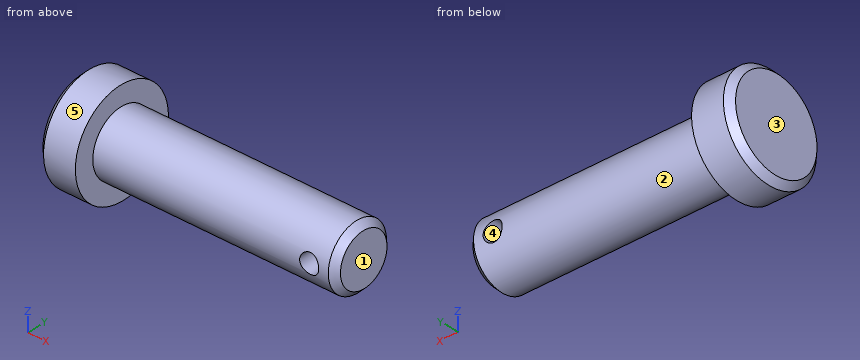
```python
from build123d import *

# Parameters (mm, degrees)
CHAMFER_1_SIZE           = 1
CHAMFER_2_SIZE           = 1
CUT_EXTRUDE_2_DEPTH      = 29.599611497
CUT_EXTRUDE_2_DEPTH_BACK = 29.599611497
SKETCH_2_R               = 1.5


with BuildPart() as part:
    # 草图1 → 旋转1 (revolve)
    with BuildSketch(Plane.XY, mode=Mode.PRIVATE) as revolve_1_sk:
        Polygon((-26.266666667, 0), (-26.266666667, 8), (-20.266666667, 8), (-20.266666667, 5), (17.733333333, 5), (17.733333333, 0), align=None)
    revolve(revolve_1_sk.sketch.rotate(Axis((0, 0, 0), (-1, 0, 0)), 90), axis=Axis((0, 0, 0), (-1, 0, 0)))

    # 倒角1
    chamfer_1_edges = [part.edges().sort_by_distance(p)[0] for p in [
        (17.733333333, 0, 5),
    ]]
    chamfer(chamfer_1_edges, length=CHAMFER_1_SIZE)

    # 倒角2
    chamfer_2_edges = [part.edges().sort_by_distance(p)[0] for p in [
        (-26.266666667, 0, 8),
    ]]
    chamfer(chamfer_2_edges, length=CHAMFER_2_SIZE)

    # 草图2 → 切除-拉伸2 (cut, two sides: drawn at the far end of the back side and taken through both)
    with BuildSketch(Plane(origin=(0, 0, 0), x_dir=(1, 0, 0), z_dir=(0, 1, 0)).offset(-CUT_EXTRUDE_2_DEPTH_BACK)):
        with Locations(Location((13.733333333, 0, 0), (0, 0, 270))):
            Circle(SKETCH_2_R)
    extrude(amount=CUT_EXTRUDE_2_DEPTH + CUT_EXTRUDE_2_DEPTH_BACK, mode=Mode.SUBTRACT)


solid = part.part
```
Can you work these out from the model? Positions are in its coordinate system, mm. Face numbers are marked on the shaded views. A direction names the side the tool comes from. Give positions to 0.01 mm unless a question says otherwise; leave off trailing zeros. Order: outer loops, then holes, each group sorted by start corner. A loop starts at its lowest first (then second) coordinate and runs counter-clockwise, first axis right, second up. Notation, with made-up numbers: M 11,42.5 L 60,42.5 A13 cw 60,52.5 Z; hole C -11,43.25 d10. An arc over 180 degrees is marked long. One line per item, written item: value.
1) For P1, Ø5, axis at x = 9.5, z = 1, coming from the -Y side; P2, Ø2, axis at x = 11, z = 2.5, coming from the +Y side; P3, Ø2, axis at x = -9, y = -2.5, coming from the -Z side; P4, Ø1.8, axis at x = 13.73, z = 0, coming from the -Y side, each with a flat end and sliding along its axis, tell me the tip position at first contact or that it passes through.
Answer sheet:
P1: stops at y = -5
P2: stops at y = 4.77
P3: stops at z = -4.77
P4: passes through
2) We'd pull the mould along X, two halves only. Please class the marked faces 3, 4 and 5: released by +X, released by -X, zero draft, split by the parting line, or undercut.
Answer sheet:
face 3: released by -X
face 4: undercut
face 5: zero draft
3) On a 3-axis mill with a long thin cutter (end or side, diameter ignored), from which of +Z, -Z, +X, -X, +Y, -Y can I reach the whole of each face in a straight line? I mean the marked faces 1 and 2. Say none if no direction works.
Answer sheet:
face 1: +Z, -Z, +X, +Y, -Y
face 2: +X
4) Please list where these lines run through material, in increasing order: line 1 along X through (y, z) = (0.75, 0); line 2 along X through (y, z) = (2.75, 6); line 3 along Y through (x, z) = (-4, -3).
Answer sheet:
line 1: x = -26.27 to 12.23, 15.23 to 17.73
line 2: x = -26.27 to -20.27
line 3: y = -4 to 4
5) I want a section at C-C, the plane x = -6.5. List the corners of the cut face in (y, z) for me, plus the area to 3 significant figures.
Answer sheet:
outline: C 0,0 d10
area: 78.5 mm^2
6) I want a section at A-A, the plane z = 0. List the corners of the cut face in (x, y) for me.
Answer sheet:
outline: M -26.27,-7 L -25.27,-8 L -20.27,-8 L -20.27,-5 L 12.23,-5 L 12.23,5 L -20.27,5 L -20.27,8 L -25.27,8 L -26.27,7 Z; M 15.23,-5 L 16.73,-5 L 17.73,-4 L 17.73,4 L 16.73,5 L 15.23,5 Z
7) I want a section at B-B, the plane y = 0. List the corners of the cut face in (x, z) for me.
Answer sheet:
outline: M -26.27,-7 L -25.27,-8 L -20.27,-8 L -20.27,-5 L 16.73,-5 L 17.73,-4 L 17.73,4 L 16.73,5 L -20.27,5 L -20.27,8 L -25.27,8 L -26.27,7 Z; hole C 13.73,0 d3
